Here's how the part is built. I have some questions about the finished solid (model axes, mm). Face numbers are marked on the shaded views. Coordinates: 2 decimals unless noted, no trailing zeros. Write each loop counter-clockwise with the first axis right and the second up, starting at its lowest first coordinate (ties: lowest second). Pieces come first, ordered by that corner, then holes.
(1) Thinking about a two-plate mould opening in Y: for the marked faces 1 and 2, which applies, released by +Y, released by -Y, zero draft, split by the parting line, or undercut?
(2) Please list where these lines run through material, in increasing order: probe 1 along Y at (x, z) = (173, -4.5); probe 2 along Y at (x, z) = (173, -6); probe 3 along Z at (x, y) = (237, 103.5).
(3) For pin 1 Ø10 at (y, z) = (105.5, -97) entering from +X; pin 2 Ø3 at (x, z) = (280, -86) entering from +Y; pin 3 Ø5 at (x, z) = (230.5, -242.5) entering from +Y, each with a flat end and sliding along its axis, tell me the tip position at first contact or that it passes through.
(4) Imagine slicing it at C-C, the plane z = -120. List the corners of the cut face in (x, y) for me.
(5) Imagine slicing it at B-B, the plane y = 0. List the corners of the cut face in (x, z) for me.
(6) Imagine slicing it at A-A, the plane x = 173. List the corners of the cut face in (y, z) for me.
(7) Imagine slicing it at D-D, the plane z = -312.5. List the corners of the cut face in (x, y) for me.
```python
from build123d import *


with BuildPart() as f1:
    # F0 (on Front) → F1 (revolve)
    with BuildSketch(Plane.XZ):
        with BuildLine():
            Line((0, 0), (0, -10))
            Line((0, -10), (1.5, -10))
            Line((1.5, -10), (1.5, -1.5))
            Line((1.5, -1.5), (10.565193, -1.5))
            Line((10.565193, -1.5), (24.930311, -324.676756))
            ThreePointArc((24.930311, -324.676756), (33.086612, -342.649857), (51.404171, -350))
            Line((51.404171, -350), (173, -350))
            Line((173, -350), (173, -348.5))
            Line((173, -348.5), (51.404171, -348.5))
            ThreePointArc((51.404171, -348.5), (34.123455, -341.565903), (26.428832, -324.610147))
            Line((26.428832, -324.610147), (12, 0))
            Line((12, 0), (0, 0))
        make_face()
    revolve(axis=Axis((173, 0, -349.25), (0, 0, -1)))


solid = f1.part
```
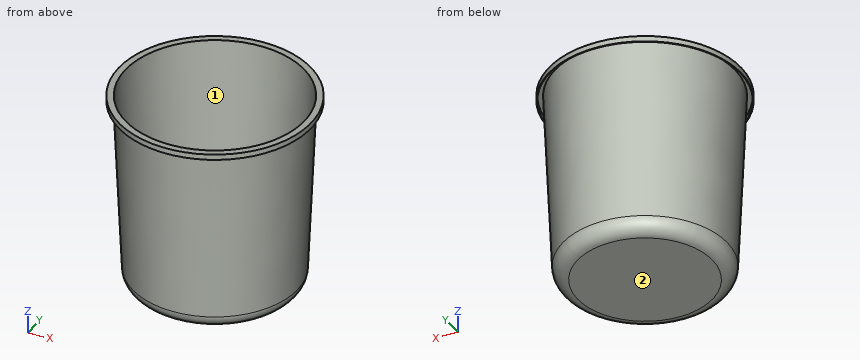
Recorded:
1. face 1: undercut
1. face 2: zero draft
2. probe 1: y = -173 to -171.5, -162.3 to -160.8, 160.8 to 162.3, 171.5 to 173
2. probe 2: y = -173 to -171.5, -162.23 to -160.73, 160.73 to 162.23, 171.5 to 173
2. probe 3: z = -350 to -348.5
3. pin 1: stops at x = 295.17
3. pin 2: stops at y = 118.53
3. pin 3: stops at y = 141.41
4. outline: circle Ø314.34 at (173, 0); hole circle Ø311.33 at (173, 0)
5. outline: (0, -10) - (1.5, -10) - (1.5, -1.5) - (10.57, -1.5) - (24.93, -324.68) arc R26.5 ccw to (51.4, -350) - (294.6, -350) arc R26.5 ccw to (321.07, -324.68) - (335.43, -1.5) - (344.5, -1.5) - (344.5, -10) - (346, -10) - (346, 0) - (334, 0) - (319.57, -324.61) arc R25 cw to (294.6, -348.5) - (51.4, -348.5) arc R25 cw to (26.43, -324.61) - (12, 0) - (0, 0) - close
6. outline: (-173, -10) - (-171.5, -10) - (-171.5, -1.5) - (-162.43, -1.5) - (-148.07, -324.68) arc R26.5 ccw to (-121.6, -350) - (121.6, -350) arc R26.5 ccw to (148.07, -324.68) - (162.43, -1.5) - (171.5, -1.5) - (171.5, -10) - (173, -10) - (173, 0) - (161, 0) - (146.57, -324.61) arc R25 cw to (121.6, -348.5) - (-121.6, -348.5) arc R25 cw to (-146.57, -324.61) - (-161, 0) - (-173, 0) - close
7. outline: circle Ø297.22 at (173, 0); hole circle Ø294.22 at (173, 0)
